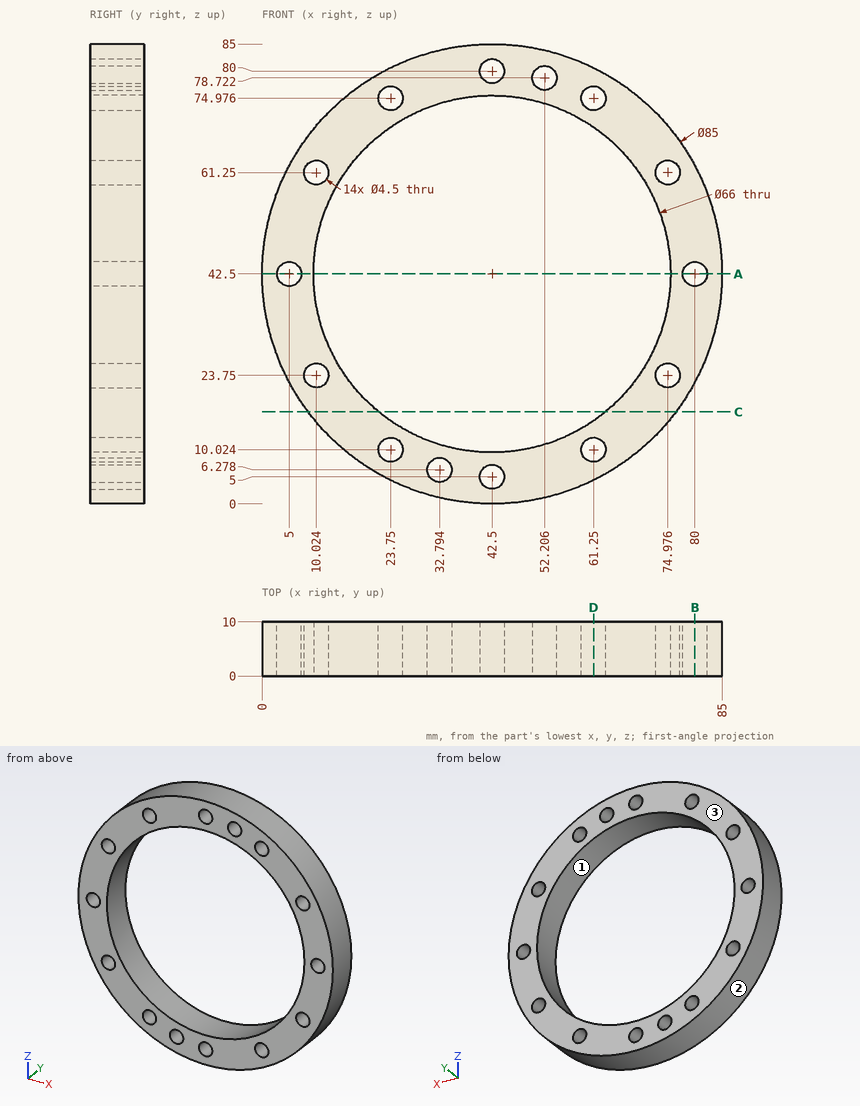
Design review of the part shown in the three views and the two pictorial views. Dimensions are in mm from the part's minimum x, y and z. Coordinates: 2 decimals unless noted, no trailing zeros. Loops run counter-clockwise (first coordinate to the right, second up) from the corner with the lowest first, then second, coordinate; pieces in that order, holes last.
Q1. We need section C-C on z = 17. State the section outline as (x, y) points, and give its area (3 significant figures).
Reported:
outline: (8.5, 0) - (21.55, 0) - (21.55, 10) - (8.5, 10) - close; (63.45, 0) - (76.5, 0) - (76.5, 10) - (63.45, 10) - close
area: 261 mm2
Q2. The part is to be moulded in two halves that separate along X. For the marked faces 1, 2 and 3, say which applies: +X half, -X half, draft (parallel to the pull), parting line (faces both ways), or undercut.
Reported:
face 1: undercut
face 2: parting line
face 3: draft
Q3. We need section D-D on x = 61.25. State the section outline as (y, z) points, and give its area (3 significant figures).
Reported:
outline: (0, 4.36) - (10, 4.36) - (10, 7.77) - (0, 7.77) - close; (0, 12.27) - (10, 12.27) - (10, 15.34) - (0, 15.34) - close; (0, 69.66) - (10, 69.66) - (10, 72.73) - (0, 72.73) - close; (0, 77.23) - (10, 77.23) - (10, 80.64) - (0, 80.64) - close
area: 130 mm2
Q4. We need section B-B on x = 80. State the section outline as (y, z) points, and give its area (3 significant figures).
Reported:
outline: (0, 22.5) - (10, 22.5) - (10, 40.25) - (0, 40.25) - close; (0, 44.75) - (10, 44.75) - (10, 62.5) - (0, 62.5) - close
area: 355 mm2
Q5. For pin 1 (3.5 mm diameter, centred on x = 61.25, z = 10.02, fed in from +Y); pin 2 (3 mm diameter, centred on y = 5, z = 52.5, fed in from +X), all flat-tipped, find the tip position at first contact; note any pin that passes through.
Reported:
pin 1: passes through
pin 2: stops at x = 84.14
Q6. To check wall thickness, follow line 1 (Z direction, x = 41, y = 3) (1 decimal); line 2 (Z direction, x = 8.5, y = 6.25) (1 decimal); line 3 (Z direction, x = 42.5, y = 2). State the ranges of each line that lie inside material, in increasing order.
Reported:
line 1: z = 0 to 3.3, 6.7 to 9.5, 75.5 to 78.3, 81.7 to 85
line 2: z = 17 to 22.1, 25.4 to 59.6, 62.9 to 68
line 3: z = 0 to 2.75, 7.25 to 9.5, 75.5 to 77.75, 82.25 to 85
Q7. We need section A-A on z = 42.5. State the section outline as (x, y) points.
Reported:
outline: (0, 0) - (2.75, 0) - (2.75, 10) - (0, 10) - close; (7.25, 0) - (9.5, 0) - (9.5, 10) - (7.25, 10) - close; (75.5, 0) - (77.75, 0) - (77.75, 10) - (75.5, 10) - close; (82.25, 0) - (85, 0) - (85, 10) - (82.25, 10) - close
